```python
from build123d import *

# Parameters (mm, degrees)
SKETCH_1_R          = 3.5
SKETCH_1_R_2        = 4
EXTRUDE_1_DEPTH     = 30
SKETCH_3_R          = 10
CUT_EXTRUDE_1_DEPTH = 77.234252505


with BuildPart() as part:
    # Эскиз1 → Бобышка-Вытянуть1 (new body)
    # profile 1 of 7: a face of its own
    with BuildSketch(Plane.XY):
        with BuildLine():
            Line((40.454647664, 45.906660544), (-9.858796034, 17.401268367))
            ThreePointArc((-9.858796034, 17.401268367), (10.070354495, 17.279697924), (20, 0))
            ThreePointArc((20, 0), (19.339407531, -5.097775626), (17.401268367, -9.858796034))
            Line((17.401268367, -9.858796034), (45.906660544, 40.454647664))
            ThreePointArc((45.906660544, 40.454647664), (39.597979746, 39.597979746), (40.454647664, 45.906660544))
        make_face()
    # profile 2 of 7: a face of its own
    with BuildSketch(Plane.XY):
        with BuildLine():
            ThreePointArc((20, 0), (10.070354495, 17.279697924), (-9.858796034, 17.401268367))
            ThreePointArc((-9.858796034, 17.401268367), (-19.957067928, -1.309747955), (-7.5, -18.540496218))
            Line((-7.5, -18.540496218), (-7.5, 0))
            ThreePointArc((-7.5, 0), (0, 7.5), (7.5, 0))
            Line((7.5, 0), (7.5, -18.540496218))
            ThreePointArc((7.5, -18.540496218), (13.185646404, -15.037909726), (17.401268367, -9.858796034))
            ThreePointArc((17.401268367, -9.858796034), (19.339407531, -5.097775626), (20, 0))
        make_face()
    # profile 3 of 7: a face of its own
    with BuildSketch(Plane.XY):
        with BuildLine():
            Line((-7.5, 0), (-7.5, -18.540496218))
            ThreePointArc((-7.5, -18.540496218), (0, -20), (7.5, -18.540496218))
            Line((7.5, -18.540496218), (7.5, 0))
            ThreePointArc((7.5, 0), (0, 7.5), (-7.5, 0))
        make_face()
    # profile 4 of 7: a face of its own
    with BuildSketch(Plane.XY):
        with BuildLine():
            ThreePointArc((20, 0), (10.070354495, 17.279697924), (-9.858796034, 17.401268367))
            ThreePointArc((-9.858796034, 17.401268367), (-19.957067928, -1.309747955), (-7.5, -18.540496218))
            Line((-7.5, -18.540496218), (-7.5, 0))
            ThreePointArc((-7.5, 0), (0, 7.5), (7.5, 0))
            Line((7.5, 0), (7.5, -18.540496218))
            ThreePointArc((7.5, -18.540496218), (13.185646404, -15.037909726), (17.401268367, -9.858796034))
            ThreePointArc((17.401268367, -9.858796034), (19.339407531, -5.097775626), (20, 0))
        make_face()
    # profile 5 of 7: a face of its own
    with BuildSketch(Plane.XY):
        with BuildLine():
            Line((-7.5, 0), (-7.5, -18.540496218))
            ThreePointArc((-7.5, -18.540496218), (0, -20), (7.5, -18.540496218))
            Line((7.5, -18.540496218), (7.5, 0))
            ThreePointArc((7.5, 0), (0, 7.5), (-7.5, 0))
        make_face()
    # profile 6 of 7: a face of its own
    with BuildSketch(Plane.XY):
        with BuildLine():
            ThreePointArc((7.5, -18.540496218), (0, -20), (-7.5, -18.540496218))
            Line((-7.5, -18.540496218), (-7.5, -45))
            ThreePointArc((-7.5, -45), (0, -52.5), (7.5, -45))
            Line((7.5, -45), (7.5, -18.540496218))
        make_face()
        with Locations((0, -45)):
            Circle(SKETCH_1_R, mode=Mode.SUBTRACT)
    # profile 7 of 7: a face of its own
    with BuildSketch(Plane.XY):
        with Locations((42.426406871, 42.426406871)):
            Circle(SKETCH_1_R_2)
    extrude(amount=EXTRUDE_1_DEPTH)

    # Эскиз3 → Вырез-Вытянуть1 (cut, through all)
    with BuildSketch(Plane.XY.offset(30)):
        Circle(SKETCH_3_R)
        with BuildLine():
            Line((27.930717857, 31.466251763), (39.244426356, 42.779960262))
            ThreePointArc((39.244426356, 42.779960262), (42.779960262, 42.779960262), (42.779960262, 39.244426356))
            Line((42.779960262, 39.244426356), (31.466251763, 27.930717857))
            ThreePointArc((31.466251763, 27.930717857), (27.930717857, 27.930717857), (27.930717857, 31.466251763))
        make_face()
    extrude(amount=-CUT_EXTRUDE_1_DEPTH, mode=Mode.SUBTRACT)


solid = part.part
```
The listing builds one solid part. Answer for the finished solid, in the listing's coordinates (mm). A direction names the side the tool comes from. Give positions to 0.01 mm unless a question says otherwise; leave off trailing zeros. Loops run counter-clockwise (first coordinate to the right, second up) from the corner with the lowest first, then second, coordinate; pieces in that order, holes last. Notation, with made-up numbers: M 18,-36.75 L 34,-36.75 A22 ccw 34,-2.75 Z; hole C -14,25 d4. An arc over 180 degrees is marked long. One line per item, written item: value.
Q1. A cutting plane is placed at D-D on x = 41.5. Determine the outline of the cut face in (y, z), then the cut area to 3 significant figures.
Working result:
outline: M 32.68,0 L 37.96,0 L 37.96,30 L 32.68,30 Z; M 43.46,0 L 46.32,0 L 46.32,30 L 43.46,30 Z
area: 244 mm^2
Q2. Flat-ended cylindrical pins translate along their axes: P1, Ø13, axis at y = -31.5, z = 11, coming from the -X side; P2, Ø2, axis at y = -35, z = 19, coming from the +X side; P3, Ø5.5, axis at x = 0, y = -45, coming from the +Z side; P4, Ø5, axis at x = 8.5, z = 16.5, coming from the +Y side. Find the tip coordinate at first contact, or state that the pin passes through.
Working result:
P1: stops at x = -7.5
P2: stops at x = 7.5
P3: passes through
P4: stops at y = 29.22
Q3. For faces 1 (the face through (7.5, -32, 15)), 2 (the face through (-7.5, -32, 15)), 3 (the face through (37.202, 33.667, 15.21)), determine the directions among +Z, -Z, +X, -X, +Y, -Y from which every point of the face is accessible in a straight line to the end or side of a thin tool.
Working result:
face 1: +Z, -Z, +X, -Y
face 2: +Z, -Z, -X, -Y
face 3: +Z, -Z
Q4. A cutting plane is placed at B-B on x = 0. Determine the outline of the cut face in (y, z).
Working result:
outline: M -52.5,0 L -48.5,0 L -48.5,30 L -52.5,30 Z; M -41.5,0 L -10,0 L -10,30 L -41.5,30 Z; M 10,0 L 22.99,0 L 22.99,30 L 10,30 Z
Q5. Find the intervals of material crossed by line 1 (Y direction, x = 0, z = 7.5); line 2 (Y direction, x = 34.5, z = 19.25); line 3 (X direction, y = -42, z = 3.25), in increasing order. Write a range as from..to.
Working result:
line 1: y = -52.5..-48.5, -41.5..-10, 10..22.99
line 2: y = 20.32..30.96, 38.04..42.53
line 3: x = -7.5..-1.8, 1.8..7.5
Q6. A cutting plane is placed at A-A on z = 20.5. Determine the outline of the cut face in (x, y), then the cut area to 3 significant figures.
Working result:
outline: M -9.86,17.4 A20 ccw -7.5,-18.54 L -7.5,-45 A7.5 ccw 7.5,-45 L 7.5,-18.54 A20 ccw 17.4,-9.86 L 45.91,40.45 A4 ccw 40.45,45.91 Z; hole C 0,0 d20; hole C 0,-45 d7; hole M 27.93,31.47 A2.5 ccw 31.47,27.93 L 42.78,39.24 A2.5 ccw 39.24,42.78 Z
area: 2,160 mm^2
Q7. A cutting plane is placed at C-C on y = 0. Determine the outline of the cut face in (x, z), then the cut area to 3 significant figures.
Working result:
outline: M -20,0 L -10,0 L -10,30 L -20,30 Z; M 10,0 L 22.99,0 L 22.99,30 L 10,30 Z
area: 690 mm^2
